Design review of the part built by this model. Coordinates are the model's own, in mm. A direction names the side the tool comes from. Coordinates: 2 decimals unless noted, no trailing zeros. Loops run counter-clockwise (first coordinate to the right, second up) from the corner with the lowest first, then second, coordinate; pieces in that order, holes last. Notation, with made-up numbers: (-39.75, -22) -> (-9.75, -22) arc R13 cw to (-9.75, -6) -> close; hole circle Ø4 at (86.25, 35.5). An arc over 180 degrees is marked (long way). Use CSV: the item, a comma, the result in double quotes.
```python
from build123d import *

# Parameters (mm, degrees)
SKETCH1_R           = 2.032
BOSS_EXTRUDE1_DEPTH = 25.4
SKETCH5_R           = 2.286
BOSS_EXTRUDE2_DEPTH = 19.05
SKETCH2_R           = 2.286
CUT_EXTRUDE1_DEPTH  = 77.793005053
CUT_EXTRUDE2_START  = 5.55625
CUT_EXTRUDE2_DEPTH  = 7.14375
CUT_EXTRUDE3_DEPTH  = 73.955945611


with BuildPart() as part:
    # Sketch1 → Boss-Extrude1 (new, symmetric)
    with BuildSketch(Plane(origin=(0, 0, 0), x_dir=(1, 0, 0), z_dir=(0, 1, 0))):
        with BuildLine():
            Line((0, 4.7625), (-63.5, 4.7625))
            Line((-63.5, 4.7625), (-63.5, -4.7625))
            Line((-63.5, -4.7625), (0, -4.7625))
            ThreePointArc((0, -4.7625), (4.7625, 0), (0, 4.7625))
        make_face()
        with Locations(Location((0, 0, 0), (0, 0, 270))):
            Circle(SKETCH1_R, mode=Mode.SUBTRACT)
    extrude(amount=BOSS_EXTRUDE1_DEPTH, both=True)

    # Sketch5 → Boss-Extrude2 (add)
    with BuildSketch(Plane(origin=(0, -25.4, 0), x_dir=(1, 0, 0), z_dir=(0, 1, 0))):
        with BuildLine():
            Line((-23.8125, 25.4), (-23.8125, 4.7625))
            Line((-23.8125, 4.7625), (-14.2875, 4.7625))
            Line((-14.2875, 4.7625), (-14.2875, 25.4))
            ThreePointArc((-14.2875, 25.4), (-19.05, 30.1625), (-23.8125, 25.4))
        make_face()
        with Locations(Location((-19.05, 25.4, 0), (0, 0, 90))):
            Circle(SKETCH5_R, mode=Mode.SUBTRACT)
    extrude(amount=BOSS_EXTRUDE2_DEPTH)

    # Sketch2 → Cut-Extrude1 (cut, through all)
    with BuildSketch(Plane.XY.offset(4.7625)):
        with Locations((-57.15, -19.05)):
            Circle(SKETCH2_R)
    extrude(amount=-CUT_EXTRUDE1_DEPTH, mode=Mode.SUBTRACT)

    # Sketch3 → Cut-Extrude2 (cut)
    with BuildSketch(Plane(origin=(0, -25.4, 0), x_dir=(1, 0, 0), z_dir=(0, 1, 0)).offset(CUT_EXTRUDE2_START)):
        with BuildLine():
            Line((-22.225, 19.900738686), (-14.2875, 15.318020924))
            Line((-14.2875, 15.318020924), (-14.2875, 25.4))
            ThreePointArc((-14.2875, 25.4), (-19.05, 30.1625), (-23.8125, 25.4))
            Line((-23.8125, 25.4), (-23.8125, 21.199869794))
            ThreePointArc((-23.8125, 21.199869794), (-23.071555914, 20.485776966), (-22.225, 19.900738686))
        make_face()
    extrude(amount=CUT_EXTRUDE2_DEPTH, mode=Mode.SUBTRACT)

    # Sketch4 → Cut-Extrude3 (cut, through all)
    with BuildSketch(Plane(origin=(0, 0, -4.7625), x_dir=(-1, 0, 0), z_dir=(0, 0, -1))):
        Polygon((12.7, 25.4), (63.5, -15.875), (63.5, 25.4), align=None)
    extrude(amount=-CUT_EXTRUDE3_DEPTH, mode=Mode.SUBTRACT)


solid = part.part
```
Item 1: Draft analysis for pull direction Y (two halves, no side actions). For faces 1 (the face through (-22, -25.4, -5)), 2 (the face through (-59.434, -18.949, 0.067)), 3 (the face through (-18.95, -9.57, -30.16)), 4 (the face through (-4, 25.4, 0)), state which applies: pulls with the +Y half, pulls with the -Y half, needs draft (parallel to the pull), parting line crosses it, or undercut.
Checked values:
face 1,"pulls with the -Y half"
face 2,"undercut"
face 3,"needs draft"
face 4,"pulls with the +Y half"
Item 2: Clearance check with flat-ended pins moving along their axes: pin 1 (3 mm diameter, centred on y = -4, z = -11.5, fed in from -X); pin 2 (6 mm diameter, centred on x = -57.15, y = -19.05, fed in from -Z); pin 3 (5 mm diameter, centred on x = -20, z = -21, fed in from +Y); pin 4 (5.5 mm diameter, centred on y = -18.5, z = -20, fed in from -X). State where each tip first meets the part, or that it passes through.
Checked values:
pin 1,"through"
pin 2,"z = -4.76"
pin 3,"y = -6.35"
pin 4,"x = -23.81"
Item 3: Add section D-D (x = -57.15). Give the boundary of the cut face in (y, z).
Checked values:
outline,"(-25.4, -4.76) -> (-21.34, -4.76) -> (-21.34, 4.76) -> (-25.4, 4.76) -> close; (-16.76, -4.76) -> (-10.72, -4.76) -> (-10.72, 4.76) -> (-16.76, 4.76) -> close"
Item 4: Add section C-C (x = -19.05). Give the boundary of the cut face in (y, z).
Checked values:
outline,"(-25.4, -30.16) -> (-19.84, -30.16) -> (-19.84, -27.69) -> (-25.4, -27.69) -> close; (-25.4, -23.11) -> (-19.84, -23.11) -> (-19.84, -18.07) -> (-12.7, -18.07) -> (-12.7, -23.11) -> (-6.35, -23.11) -> (-6.35, -4.76) -> (20.24, -4.76) -> (20.24, 4.76) -> (-25.4, 4.76) -> close; (-12.7, -30.16) -> (-6.35, -30.16) -> (-6.35, -27.69) -> (-12.7, -27.69) -> close"
Item 5: Add section A-A (z = 0). State how many separate pieces and enclosed holes the cut face has, then the cut area to 3 significant figures.
Checked values:
separate pieces,"2"
enclosed holes,"1"
area,"2,200 mm^2"
Item 6: Machinability: for faces 5 (the face through (-19.1, -19.844, -22.8)), 6 (the face through (-19, -6.35, -18)), 7 (the face through (-23.812, -16, -15)), 8 (the face through (-14.288, -16, -15)), 9 (the face through (-63.5, -21, 0)), which of the approach directions +Z, -Z, +X, -X, +Y, -Y give a long, thin tool a straight path to every point of the face, cutting with its end or side? Answer none if there is none.
Checked values:
face 5,"-Z, +X"
face 6,"-Z, +X, -X, +Y"
face 7,"-Z, -X, +Y, -Y"
face 8,"-Z, +X, +Y, -Y"
face 9,"+Z, -Z, -X, +Y, -Y"
Item 7: Add section B-B (y = -4.5). Give the boundary of the cut face in (x, z) (1 decimal), then the cut area to 3 significant figures.
Checked values:
outline,"(-49.5, -4.8) -> (0, -4.8) arc R4.8 ccw to (0, 4.8) -> (-49.5, 4.8) -> close; hole circle Ø4.1 at (0, 0)"
area,"494 mm^2"
Item 8: To check wall thickness, follow line 1 along X through (y, z) = (-22.6, -25.4); line 2 along X through (y, z) = (-20, -16); line 3 along Z through (x, y) = (-8, 18.5). State the ranges of each line that lie inside material, in increasing order.
Checked values:
line 1,"-23.81 to -21.34, -16.76 to -14.29"
line 2,"-23.81 to -14.29"
line 3,"-4.76 to 4.76"
